```python
from build123d import *

# Parameters (mm, degrees)
CROQUIS2_R              = 1.59
CROQUIS2_R_2            = 1.5875
CROQUIS2_R_3            = 1.590000003
CROQUIS2_R_4            = 1.52
CROQUIS2_W              = 2.3
CROQUIS2_H              = 5
SALIENTE_EXTRUIR1_DEPTH = 2


with BuildPart() as part:
    # Croquis2 → Saliente-Extruir1 (new body)
    with BuildSketch(Plane(origin=(0, 0, 0), x_dir=(1, 0, 0), z_dir=(0, 1, 0))):
        with BuildLine():
            Line((-18.25536195, -12.016111847), (-25.654088229, -20.470893156))
            ThreePointArc((-25.654088229, -20.470893156), (-26.519678095, -22.835784768), (-25.57354606, -25.169621165))
            Line((-25.57354606, -25.169621165), (-24.742372568, -25.914075676))
            Line((-24.742372568, -25.914075676), (-22.972153409, -27.446083615))
            ThreePointArc((-22.972153409, -27.446083615), (-20.975135837, -28.097582379), (-18.96479715, -27.488428717))
            ThreePointArc((-18.96479715, -27.488428717), (-17.537304596, -26.067045976), (-15.541615973, -25.792654271))
            Line((-15.541615973, -25.792654271), (-9.856067815, -20.097418653))
            ThreePointArc((-9.856067815, -20.097418653), (-7.911909666, -18.801779306), (-5.620288821, -18.346909954))
            Line((-5.620288821, -18.346909954), (5.620288821, -18.346909954))
            ThreePointArc((5.620288821, -18.346909954), (7.911909666, -18.801779306), (9.856067815, -20.097418653))
            Line((9.856067815, -20.097418653), (15.541615973, -25.792654271))
            ThreePointArc((15.541615973, -25.792654271), (17.537304596, -26.067045976), (18.96479715, -27.488428717))
            ThreePointArc((18.96479715, -27.488428717), (20.975135837, -28.097582379), (22.972153409, -27.446083615))
            Line((22.972153409, -27.446083615), (24.742372568, -25.914075676))
            Line((24.742372568, -25.914075676), (25.57354606, -25.169621165))
            ThreePointArc((25.57354606, -25.169621165), (26.519678095, -22.835784768), (25.654088229, -20.470893156))
            Line((25.654088229, -20.470893156), (18.25536195, -12.016111847))
            ThreePointArc((18.25536195, -12.016111847), (16.419845193, -8.948181441), (15.780779256, -5.4306662))
            Line((15.780779256, -5.4306662), (15.780779256, 5.4306662))
            ThreePointArc((15.780779256, 5.4306662), (16.419845193, 8.948181441), (18.25536195, 12.016111847))
            Line((18.25536195, 12.016111847), (25.654088229, 20.470893156))
            ThreePointArc((25.654088229, 20.470893156), (26.530308227, 23.005689388), (25.355142951, 25.416485937))
            Line((25.355142951, 25.416485937), (18.78888202, 30.200247321))
            ThreePointArc((18.78888202, 30.200247321), (17.806953387, 31.422484528), (16.34255947, 31.982482822))
            Line((16.34255947, 31.982482822), (12.561458087, 34.737153551))
            ThreePointArc((12.561458087, 34.737153551), (9.874030074, 35.155779391), (8.394864944, 32.873327323))
            Line((8.394864944, 32.873327323), (8.021421807, 31.657286053))
            ThreePointArc((8.021421807, 31.657286053), (7.691575606, 30.205895283), (7.580808922, 28.721622928))
            Line((7.580808922, 28.721622928), (7.580808922, 25.398403441))
            ThreePointArc((7.580808922, 25.398403441), (7.695379905, 23.889001856), (8.036467551, 22.414186995))
            Line((8.036467551, 22.414186995), (8.38479276, 21.300147594))
            ThreePointArc((8.38479276, 21.300147594), (7.968360691, 20.527060023), (7.14619906, 20.218627998))
            Line((7.14619906, 20.218627998), (6.412176591, 20.218627998))
            ThreePointArc((6.412176591, 20.218627998), (5.70506981, 20.511521217), (5.412176591, 21.218627998))
            Line((5.412176591, 21.218627998), (5.412176591, 22.079422133))
            ThreePointArc((5.412176591, 22.079422133), (5.308230514, 23.093648922), (5.000714199, 24.065705754))
            Line((5.000714199, 24.065705754), (2.518171143, 29.800658234))
            ThreePointArc((2.518171143, 29.800658234), (1.464464231, 30.91120601), (0, 31.357254366))
            ThreePointArc((0, 31.357254366), (-1.464464231, 30.91120601), (-2.518171143, 29.800658234))
            Line((-2.518171143, 29.800658234), (-5.000714199, 24.065705754))
            ThreePointArc((-5.000714199, 24.065705754), (-5.308230514, 23.093648922), (-5.412176591, 22.079422133))
            Line((-5.412176591, 22.079422133), (-5.412176591, 21.218627998))
            ThreePointArc((-5.412176591, 21.218627998), (-5.70506981, 20.511521217), (-6.412176591, 20.218627998))
            Line((-6.412176591, 20.218627998), (-7.14619906, 20.218627998))
            ThreePointArc((-7.14619906, 20.218627998), (-7.968360691, 20.527060023), (-8.38479276, 21.300147594))
            Line((-8.38479276, 21.300147594), (-8.036467551, 22.414186995))
            ThreePointArc((-8.036467551, 22.414186995), (-7.695379905, 23.889001856), (-7.580808922, 25.398403441))
            Line((-7.580808922, 25.398403441), (-7.580808922, 28.721622928))
            ThreePointArc((-7.580808922, 28.721622928), (-7.691575606, 30.205895283), (-8.021421807, 31.657286053))
            Line((-8.021421807, 31.657286053), (-8.394864944, 32.873327323))
            ThreePointArc((-8.394864944, 32.873327323), (-9.874030074, 35.155779391), (-12.561458087, 34.737153551))
            Line((-12.561458087, 34.737153551), (-16.34255947, 31.982482822))
            ThreePointArc((-16.34255947, 31.982482822), (-17.806953387, 31.422484528), (-18.78888202, 30.200247321))
            Line((-18.78888202, 30.200247321), (-25.355142951, 25.416485937))
            ThreePointArc((-25.355142951, 25.416485937), (-26.530308227, 23.005689388), (-25.654088229, 20.470893156))
            Line((-25.654088229, 20.470893156), (-18.25536195, 12.016111847))
            ThreePointArc((-18.25536195, 12.016111847), (-16.419845193, 8.948181441), (-15.780779256, 5.4306662))
            Line((-15.780779256, 5.4306662), (-15.780779256, -5.4306662))
            ThreePointArc((-15.780779256, -5.4306662), (-16.419845193, -8.948181441), (-18.25536195, -12.016111847))
        make_face()
        with Locations(Location((-15.25, 15.25, 0), (0, 0, 270))):
            Circle(CROQUIS2_R, mode=Mode.SUBTRACT)
        with Locations(Location((-20.475551104, 22.857961383, 0), (0, 0, 270))):
            Circle(CROQUIS2_R_2, mode=Mode.SUBTRACT)
        with Locations(Location((-16.040434505, 28.997734842, 0), (0, 0, 270))):
            Circle(CROQUIS2_R_2, mode=Mode.SUBTRACT)
        with Locations(Location((15.25, 15.25, 0), (0, 0, 270))):
            Circle(CROQUIS2_R, mode=Mode.SUBTRACT)
        with Locations(Location((20.565117485, -22.768131206, 0), (0, 0, 270))):
            Circle(CROQUIS2_R_2, mode=Mode.SUBTRACT)
        with Locations(Location((-20.341013705, -22.888433679, 0), (0, 0, 270))):
            Circle(CROQUIS2_R_2, mode=Mode.SUBTRACT)
        with Locations(Location((-15.160301721, -15.249868102, 0), (0, 0, 270))):
            Circle(CROQUIS2_R_3, mode=Mode.SUBTRACT)
        with Locations(Location((15.339566381, -15.160169822, 0), (0, 0, 270))):
            Circle(CROQUIS2_R_2, mode=Mode.SUBTRACT)
        with Locations(Location((20.430580086, 22.978263857, 0), (0, 0, 270))):
            Circle(CROQUIS2_R_2, mode=Mode.SUBTRACT)
        with Locations(Location((15.959427109, 29.091844512, 0), (0, 0, 270))):
            Circle(CROQUIS2_R_4, mode=Mode.SUBTRACT)
        with BuildLine():
            Line((-1.35, 8.308113143), (-1.35, 5.718277528))
            ThreePointArc((-1.35, 5.718277528), (0, 4.368277528), (1.35, 5.718277528))
            Line((1.35, 5.718277528), (1.35, 8.308113143))
            ThreePointArc((1.35, 8.308113143), (0, 9.658113143), (-1.35, 8.308113143))
        make_face(mode=Mode.SUBTRACT)
        with BuildLine():
            Line((-7.808878773, -5.814643086), (-7.808878773, -3.761226184))
            ThreePointArc((-7.808878773, -3.761226184), (-9.158878773, -2.411226184), (-10.508878773, -3.761226184))
            Line((-10.508878773, -3.761226184), (-10.508878773, -5.814643086))
            ThreePointArc((-10.508878773, -5.814643086), (-9.158878773, -7.164643086), (-7.808878773, -5.814643086))
        make_face(mode=Mode.SUBTRACT)
        with BuildLine():
            Line((-2.890898672, -4.911820136), (-2.890898672, -3.666330657))
            ThreePointArc((-2.890898672, -3.666330657), (-4.240898672, -2.316330657), (-5.590898672, -3.666330657))
            Line((-5.590898672, -3.666330657), (-5.590898672, -4.911820136))
            ThreePointArc((-5.590898672, -4.911820136), (-4.240898672, -6.261820136), (-2.890898672, -4.911820136))
        make_face(mode=Mode.SUBTRACT)
        with BuildLine():
            Line((8.19090575, -6.317028248), (8.19090575, -4.263611346))
            ThreePointArc((8.19090575, -4.263611346), (9.54090575, -2.913611346), (10.89090575, -4.263611346))
            Line((10.89090575, -4.263611346), (10.89090575, -6.317028248))
            ThreePointArc((10.89090575, -6.317028248), (9.54090575, -7.667028248), (8.19090575, -6.317028248))
        make_face(mode=Mode.SUBTRACT)
        with BuildLine():
            Line((3.27292565, -4.911820136), (3.27292565, -4.074486775))
            ThreePointArc((3.27292565, -4.074486775), (4.62292565, -2.724486775), (5.97292565, -4.074486775))
            Line((5.97292565, -4.074486775), (5.97292565, -4.911820136))
            ThreePointArc((5.97292565, -4.911820136), (4.62292565, -6.261820136), (3.27292565, -4.911820136))
        make_face(mode=Mode.SUBTRACT)
        with Locations((-10.694064619, 27.741630955)):
            Rectangle(CROQUIS2_W, CROQUIS2_H, mode=Mode.SUBTRACT)
        with BuildLine():
            Line((-1.35, -7.377770249), (-1.35, -4.787934635))
            ThreePointArc((-1.35, -4.787934635), (0, -3.437934635), (1.35, -4.787934635))
            Line((1.35, -4.787934635), (1.35, -7.377770249))
            ThreePointArc((1.35, -7.377770249), (0, -8.727770249), (-1.35, -7.377770249))
        make_face(mode=Mode.SUBTRACT)
        with BuildLine():
            Line((0.235062276, 12.522369289), (-0.235062276, 12.522369289))
            ThreePointArc((-0.235062276, 12.522369289), (-2.488062555, 13.552617925), (-3.182517958, 15.930674736))
            Line((-3.182517958, 15.930674736), (-1.97907978, 24.185590314))
            ThreePointArc((-1.97907978, 24.185590314), (0, 25.897071292), (1.97907978, 24.185590314))
            Line((1.97907978, 24.185590314), (3.182517958, 15.930674736))
            ThreePointArc((3.182517958, 15.930674736), (2.488062555, 13.552617925), (0.235062276, 12.522369289))
        make_face(mode=Mode.SUBTRACT)
        with Locations((10.694064619, 27.741630955)):
            Rectangle(CROQUIS2_W, CROQUIS2_H, mode=Mode.SUBTRACT)
        with BuildLine():
            Line((3.27292565, 5.84216303), (3.27292565, 5.004829668))
            ThreePointArc((3.27292565, 5.004829668), (4.62292565, 3.654829668), (5.97292565, 5.004829668))
            Line((5.97292565, 5.004829668), (5.97292565, 5.84216303))
            ThreePointArc((5.97292565, 5.84216303), (4.62292565, 7.19216303), (3.27292565, 5.84216303))
        make_face(mode=Mode.SUBTRACT)
        with BuildLine():
            Line((8.19090575, 7.247371142), (8.19090575, 5.19395424))
            ThreePointArc((8.19090575, 5.19395424), (9.54090575, 3.84395424), (10.89090575, 5.19395424))
            Line((10.89090575, 5.19395424), (10.89090575, 7.247371142))
            ThreePointArc((10.89090575, 7.247371142), (9.54090575, 8.597371142), (8.19090575, 7.247371142))
        make_face(mode=Mode.SUBTRACT)
        with BuildLine():
            Line((-2.890898672, 5.84216303), (-2.890898672, 4.596673551))
            ThreePointArc((-2.890898672, 4.596673551), (-4.240898672, 3.246673551), (-5.590898672, 4.596673551))
            Line((-5.590898672, 4.596673551), (-5.590898672, 5.84216303))
            ThreePointArc((-5.590898672, 5.84216303), (-4.240898672, 7.19216303), (-2.890898672, 5.84216303))
        make_face(mode=Mode.SUBTRACT)
        with BuildLine():
            Line((-7.808878773, 6.744985979), (-7.808878773, 4.691569078))
            ThreePointArc((-7.808878773, 4.691569078), (-9.158878773, 3.341569078), (-10.508878773, 4.691569078))
            Line((-10.508878773, 4.691569078), (-10.508878773, 6.744985979))
            ThreePointArc((-10.508878773, 6.744985979), (-9.158878773, 8.094985979), (-7.808878773, 6.744985979))
        make_face(mode=Mode.SUBTRACT)
    extrude(amount=SALIENTE_EXTRUIR1_DEPTH)


solid = part.part
```
Model file for the job. Use its own axes, mm. A direction names the side the tool comes from. Coordinates: 2 decimals unless noted, no trailing zeros. Loops run counter-clockwise (first coordinate to the right, second up) from the corner with the lowest first, then second, coordinate; pieces in that order, holes last. Notation, with made-up numbers: (59, 5) - (78, 5) arc R12 ccw to (78, 14) - close; hole circle Ø3 at (-30.5, 41.25). An arc over 180 degrees is marked (long way). Write item = value, one per line. Start each with the question number.
Item 1: 3-axis set-ups, long thin cutter, end or side, ignore diameter. For faces 1 (the face through (16.44, 0.99, 9)), 2 (the face through (-21.9, 0.99, 16.18)), 3 (the face through (-9.13, 0.99, -3.34)), 4 (the face through (-7.581, 1, -27)), 5 (the face through (12.659, 0.986, 22.905)): which of +Z, -Z, +X, -X, +Y, -Y reach the whole face in a straight line?
Item 2: Drop flat-ended pins along their axis: pin 1 Ø5 at (x, z) = (-16.04, -29) entering from +Y; pin 2 Ø2.5 at (x, z) = (20.57, 22.77) entering from +Y; pin 3 Ø0.7 at (y, z) = (0.5, -21.5) entering from +X; pin 4 Ø0.7 at (y, z) = (1.5, -21.5) entering from -X. Give the stop position or say it passes through.
Item 3: Pull direction X, two halves, no side cores. Call faces 6 (the face through (2.57, 0.99, -20.12)), 7 (the face through (14.48, 0.99, -33.34)), 8 (the face through (-23.87, 0.99, 26.67)): +X half, -X half, draft (parallel to the pull), parting line (faces both ways), or undercut.
Item 4: Saw through at A-A, the plane z = -15.25. List the corners of the cut face in (x, y).
Item 5: Saw through at B-B, the plane z = 14.5. List the corners of the cut face in (x, y).
Item 6: Wall check: probe 1 along X at (y, z) = (0.3, 5); probe 2 along X at (y, z) = (1.85, 15); probe 3 along X at (y, z) = (0.2, -16). Give the ranges that are in metal, low to high. Write a range as [from, to].
Item 7: Saw through at C-C, the plane y = 0.4. State how many separate pieces and enclosed holes the cut face has, then the cut area to 3 significant figures.
Answers:
q1.face_1 = +X, +Y, -Y
q1.face_2 = -X, +Y, -Y
q1.face_3 = +Y, -Y
q1.face_4 = -Z, +Y, -Y
q1.face_5 = +Z, +Y, -Y
q2.pin_1 = 2
q2.pin_2 = through
q2.pin_3 = 26.41
q2.pin_4 = -26.41
q3.face_6 = undercut
q3.face_7 = +X half
q3.face_8 = -X half
q4.outline = (-21.09, 0) - (-16.84, 0) - (-16.84, 2) - (-21.09, 2) - close; (-13.66, 0) - (-3.2, 0) - (-3.2, 2) - (-13.66, 2) - close; (3.2, 0) - (13.66, 0) - (13.66, 2) - (3.2, 2) - close; (16.84, 0) - (21.09, 0) - (21.09, 2) - (16.84, 2) - close
q5.outline = (-20.43, 0) - (-16.56, 0) - (-16.56, 2) - (-20.43, 2) - close; (-13.76, 0) - (13.9, 0) - (13.9, 2) - (-13.76, 2) - close; (16.78, 0) - (20.43, 0) - (20.43, 2) - (16.78, 2) - close
q6.probe_1 = [-15.78, -10.51], [-7.81, -5.59], [-2.89, -1.35], [1.35, 3.28], [5.97, 8.19], [10.89, 15.78]
q6.probe_2 = [-20.87, -16.73], [-13.59, 13.76], [16.92, 20.87]
q6.probe_3 = [-21.74, -16.65], [-13.85, -3.17], [3.17, 13.85], [16.65, 21.74]
q7.separate_pieces = 1
q7.enclosed_holes = 23
q7.area = 1,850 mm2
